For this review, take the finished solid that the model builds, in its own axes (mm). A direction names the side the tool comes from. Round coordinates to 2 decimals unless told otherwise and drop trailing zeros. Write each loop counter-clockwise with the first axis right and the second up, starting at its lowest first coordinate (ties: lowest second). Pieces come first, ordered by that corner, then holes. Notation, with made-up numbers: (24, 25.5) -> (47, 25.5) arc R18 ccw to (47, 36.5) -> close; hole circle Ø7 at (75.5, 74). An arc over 180 degrees is marked (long way). Answer in a Markdown table with one row per item.
from build123d import *

# Parameters (mm, degrees)
SHAPEBINDER_R       = 3.2
SHAPEBINDER_R_2     = 2.75
PAD001_DEPTH        = 19.05
HOLE002_D           = 6.4
HOLE002_CBORE_D     = 10.5
HOLE002_CBORE_DEPTH = 8
HOLE003_D           = 5.5
HOLE003_CBORE_D     = 9.5
HOLE003_CBORE_DEPTH = 6
HOLE004_D           = 6.4
HOLE004_CBORE_D     = 10.5
HOLE004_CBORE_DEPTH = 8
SKETCH021_R         = 2.1
POCKET011_DEPTH     = 19.051
SKETCH026_R         = 2.5
POCKET012_DEPTH     = 20


with BuildPart() as part:
    # ShapeBinder → Pad001 (new body)
    with BuildSketch(Plane(origin=(23.746009, 0, 109.511429), x_dir=(-1, 0, 0), z_dir=(0, -1, 0))):
        Polygon((107.746009, -167.188571), (107.746009, -2.088571), (49.746009, 83.511429), (49.746009, 131.511429), (-146.253991, 131.511429), (-146.253991, 83.511429), (24.346009, -167.188571), align=None)
        with Locations((69.646009, -129.088571)):
            Circle(SHAPEBINDER_R, mode=Mode.SUBTRACT)
        with Locations((95.046009, -129.088571)):
            Circle(SHAPEBINDER_R, mode=Mode.SUBTRACT)
        with Locations((69.646009, -40.188571)):
            Circle(SHAPEBINDER_R, mode=Mode.SUBTRACT)
        with Locations((95.046009, -40.188571)):
            Circle(SHAPEBINDER_R, mode=Mode.SUBTRACT)
        with Locations((69.646009, -14.788571)):
            Circle(SHAPEBINDER_R, mode=Mode.SUBTRACT)
        with Locations((95.046009, -14.788571)):
            Circle(SHAPEBINDER_R, mode=Mode.SUBTRACT)
        with Locations((69.646009, -154.488571)):
            Circle(SHAPEBINDER_R, mode=Mode.SUBTRACT)
        with Locations((95.046009, -154.488571)):
            Circle(SHAPEBINDER_R, mode=Mode.SUBTRACT)
        with Locations((-138.253991, 125.511429)):
            Circle(SHAPEBINDER_R_2, mode=Mode.SUBTRACT)
        with Locations((-138.253991, 93.511429)):
            Circle(SHAPEBINDER_R_2, mode=Mode.SUBTRACT)
        with Locations((5.746009, 125.511429)):
            Circle(SHAPEBINDER_R_2, mode=Mode.SUBTRACT)
        with Locations((41.746009, 125.511429)):
            Circle(SHAPEBINDER_R_2, mode=Mode.SUBTRACT)
        with Locations((5.746009, 93.511429)):
            Circle(SHAPEBINDER_R_2, mode=Mode.SUBTRACT)
        with Locations((41.746009, 93.511429)):
            Circle(SHAPEBINDER_R_2, mode=Mode.SUBTRACT)
        with Locations((-102.253991, 125.511429)):
            Circle(SHAPEBINDER_R_2, mode=Mode.SUBTRACT)
        with Locations((-102.253991, 93.511429)):
            Circle(SHAPEBINDER_R_2, mode=Mode.SUBTRACT)
    extrude(amount=PAD001_DEPTH)

    # Hole002 (through all)
    with Locations(Plane(origin=(0, 0, 0), x_dir=(-1, 0, 0), z_dir=(0, 1, 0))):
        with Locations((45.9, 238.6), (71.3, 238.6), (71.3, 149.7), (45.9, 149.7), (45.9, 124.3), (71.3, 124.3), (71.3, 264), (45.9, 264)):
            CounterBoreHole(HOLE002_D / 2, HOLE002_CBORE_D / 2, HOLE002_CBORE_DEPTH)

    # Hole003 (through all)
    with Locations(Plane(origin=(0, 0, 0), x_dir=(-1, 0, 0), z_dir=(0, 1, 0))):
        with Locations((18, -16), (-162, 16), (-162, -16), (-18, -16), (-126, -16), (-18, 16), (18, 16), (18, 16), (-126, 16)):
            CounterBoreHole(HOLE003_D / 2, HOLE003_CBORE_D / 2, HOLE003_CBORE_DEPTH)

    # Hole004 (through all)
    with Locations(Plane(origin=(0, 0, 0), x_dir=(-1, 0, 0), z_dir=(0, 1, 0))):
        with Locations((71.3, 194.15)):
            CounterBoreHole(HOLE004_D / 2, HOLE004_CBORE_D / 2, HOLE004_CBORE_DEPTH)

    # Sketch021 → Pocket011 (cut, through all)
    with BuildSketch(Plane(origin=(0, 0, 0), x_dir=(-1, 0, 0), z_dir=(0, 1, 0))):
        with Locations((-88, 16)):
            Circle(SKETCH021_R)
        with Locations((-88, -16)):
            Circle(SKETCH021_R)
        with Locations((-56, 16)):
            Circle(SKETCH021_R)
        with Locations((-56, -16)):
            Circle(SKETCH021_R)
    extrude(amount=-POCKET011_DEPTH, mode=Mode.SUBTRACT)

    # Sketch026 (on Face7 of Pocket011) → Pocket012 (cut)
    with BuildSketch(Plane(origin=(-26, 0, 0), x_dir=(0, -1, 0), z_dir=(-1, 0, 0))):
        with Locations((9.525, 0)):
            Circle(SKETCH026_R)
    extrude(amount=-POCKET012_DEPTH, mode=Mode.SUBTRACT)


with BuildPart() as part_1:
    # Body001 placement: moved
    add(part.part.moved(Location((0, 407, 0))))


solid = part_1.part
1) For line 1 (Z direction, x = 126, y = 393); line 2 (X direction, y = 396, z = 264); line 3 (Z direction, x = 54.5, y = 397.25), list the stretches that pass through material, from the lowest coordinate up. Write a range as [from, to].
Solved:
| item | result |
|---|---|
| line 1 | [-22, -18.75], [-13.25, 13.25], [18.75, 90.66] |
| line 2 | [-84, -74.5], [-68.1, -49.1], [-42.7, 8.04] |
| line 3 | [-22, -17.47], [-14.53, 14.53], [17.47, 195.73] |
2) Consider section B-B on x = -71.3. State how many separate pieces and enclosed holes the cut face has, then the cut area to 3 significant figures.
Solved:
| item | result |
|---|---|
| separate pieces | 6 |
| enclosed holes | 0 |
| area | 2,730 mm² |
3) Mouldability with a two-part tool opening along X and no side actions: class faces 3 (the flat face through (71, 398, -22)), 4 (the flat face through (-26, 395, 2)), 5 (the cylindrical face through (121.47, 404.04, -14.57)) as pulls with the +X half, pulls with the -X half, needs draft (parallel to the pull), parting line crosses it, or undercut.
Solved:
| item | result |
|---|---|
| face 3 | needs draft |
| face 4 | pulls with the -X half |
| face 5 | undercut |
4) Consider section C-C on x = 67. State the section outline as (y, z) points.
Solved:
| item | result |
|---|---|
| outline | (387.95, -22) -> (407, -22) -> (407, 177.36) -> (387.95, 177.36) -> close |
5) Clearance check with flat-ended pins moving along their axes: pin 1 Ø3 at (x, z) = (-47.5, 122) entering from +Y; pin 2 Ø3.5 at (x, z) = (18, 16) entering from +Y; pin 3 Ø3 at (x, z) = (161.5, -14) entering from +Y; pin 4 Ø1 at (x, y) = (102, 401) entering from +Z. State where each tip first meets the part, or that it passes through.
Solved:
| item | result |
|---|---|
| pin 1 | y = 399 |
| pin 2 | through |
| pin 3 | y = 401 |
| pin 4 | z = 126.66 |
6) Consider section A-A on z = 238.6. State the section outline as (x, y) points.
Solved:
| item | result |
|---|---|
| outline | (-84, 387.95) -> (-74.5, 387.95) -> (-74.5, 399) -> (-76.55, 399) -> (-76.55, 407) -> (-84, 407) -> close; (-68.1, 387.95) -> (-49.1, 387.95) -> (-49.1, 399) -> (-51.15, 399) -> (-51.15, 407) -> (-66.05, 407) -> (-66.05, 399) -> (-68.1, 399) -> close; (-42.7, 387.95) -> (25.33, 387.95) -> (25.33, 407) -> (-40.65, 407) -> (-40.65, 399) -> (-42.7, 399) -> close |
7) For faces 1 (the cylindrical face through (-47.377, 393.552, 152.539)), 2 (the cylindrical face through (-45.217, 403.056, 243.805)), list the 3-axis set-ups (+Z, -Z, +X, -X, +Y, -Y) from which the entire face can be reached by the end or side of a thin tool; tool diameter is ignored.
Solved:
| item | result |
|---|---|
| face 1 | +Y, -Y |
| face 2 | +Y |
8) Consider section D-D on z = 208. State the section outline as (x, y) points.
Solved:
| item | result |
|---|---|
| outline | (-84, 387.95) -> (46.15, 387.95) -> (46.15, 407) -> (-84, 407) -> close |
